The model under review builds one solid part; all positions refer to its coordinate system, in mm. Face numbers are marked on the shaded views. A direction names the side the tool comes from. Round coordinates to 2 decimals unless told otherwise and drop trailing zeros. Order: outer loops, then holes, each group sorted by start corner. A loop starts at its lowest first (then second) coordinate and runs counter-clockwise, first axis right, second up. Notation, with made-up numbers: M -28,-5 L 31,-5 A34 ccw 31,26 Z; hole C -9.5,78 d10. An arc over 180 degrees is marked long. Answer as a JSON object with one key per item and string values. Group by question number.
1. To check wall thickness, follow probe 1 along X at (y, z) = (-214.5, 55); probe 2 along Y at (x, z) = (47, 34.5); probe 3 along X at (y, z) = (-174.5, -2). State the ranges of each line that lie inside material, in increasing order. Write a range as [from, to].
2. Add section B-B on x = 0. State the section outline as (y, z) points, and give its area (3 significant figures).
3. Machinability: for the marked faces 4 and 5, which of the approach directions +Z, -Z, +X, -X, +Y, -Y give a long, thin tool a straight path to every point of the face, cutting with its end or side? Answer none if there is none.
4. Add section A-A on y = -116. State the section outline as (x, z) points.
5. Add section C-C on z = 0. State the section outline as (x, y) points.
6. Add section D-D on x = 47. State the section outline as (y, z) points, and give its area (3 significant figures).
7. Clearance check with flat-ended pins moving along their axes: P1, Ø3, axis at x = 8.5, y = -53.5, coming from the +Z side; P2, Ø2, axis at x = -11.5, y = -177.5, coming from the +Z side; P3, Ø10, axis at x = 18, y = -91.5, coming from the +Z side. State where each tip first meets the part, or that it passes through.
8. Mouldability with a two-part tool opening along X and no side actions: class the marked faces 1, 2 and 3 as released by +X, released by -X, zero draft, split by the parting line, or undercut.
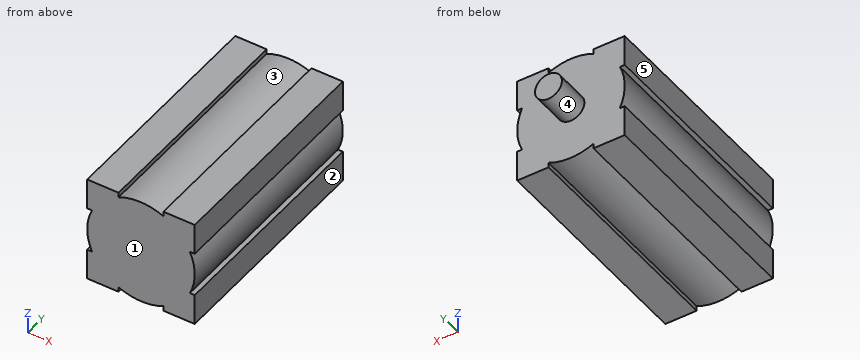
```python
from build123d import *

# Parameters (mm, degrees)
F1_DEPTH = 250
F2_R     = 15
F3_DEPTH = 38


with BuildPart() as f1:
    # F0 (on Front) → F1 (new body)
    with BuildSketch(Plane.XZ):
        with BuildLine():
            Line((-60, 25), (-54.543561, 25))
            ThreePointArc((-54.543561, 25), (-60, 0), (-54.543561, -25))
            Line((-54.543561, -25), (-60, -25))
            Line((-60, -25), (-60, -60))
            Line((-60, -60), (-25, -60))
            Line((-25, -60), (-25, -54.543561))
            ThreePointArc((-25, -54.543561), (0, -60), (25, -54.543561))
            Line((25, -54.543561), (25, -60))
            Line((25, -60), (60, -60))
            Line((60, -60), (60, -25))
            Line((60, -25), (54.543561, -25))
            ThreePointArc((54.543561, -25), (60, 0), (54.543561, 25))
            Line((54.543561, 25), (60, 25))
            Line((60, 25), (60, 60))
            Line((60, 60), (25, 60))
            Line((25, 60), (25, 54.543561))
            ThreePointArc((25, 54.543561), (0, 60), (-25, 54.543561))
            Line((-25, 54.543561), (-25, 60))
            Line((-25, 60), (-60, 60))
            Line((-60, 60), (-60, 25))
        make_face()
    extrude(amount=F1_DEPTH)

    # F2 (on face) → F3 (join)
    with BuildSketch(Plane(origin=(0, 0, 0), x_dir=(-1, 0, 0), z_dir=(0, 1, 0))):
        Circle(F2_R)
    extrude(amount=F3_DEPTH)


solid = f1.part
```
Recorded:
{
 "1": {"probe 1": "x = [-60, -25], [-23.98, 23.98], [25, 60]", "probe 2": "y = [-250, 0]", "probe 3": "x = [-59.97, 59.97]"},
 "2": {"outline": "M -250,-60 L 0,-60 L 0,-15 L 38,-15 L 38,15 L 0,15 L 0,60 L -250,60 Z", "area": "31,100 mm²"},
 "3": {"face 4": "+Y", "face 5": "+Z, -Z, -X, +Y, -Y"},
 "4": {"outline": "M -60,-60 L -25,-60 L -25,-54.54 A60 ccw 25,-54.54 L 25,-60 L 60,-60 L 60,-25 L 54.54,-25 A60 ccw 54.54,25 L 60,25 L 60,60 L 25,60 L 25,54.54 A60 ccw -25,54.54 L -25,60 L -60,60 L -60,25 L -54.54,25 A60 ccw -54.54,-25 L -60,-25 Z"},
 "5": {"outline": "M -60,-250 L 60,-250 L 60,0 L 15,0 L 15,38 L -15,38 L -15,0 L -60,0 Z"},
 "6": {"outline": "M -250,-60 L 0,-60 L 0,60 L -250,60 Z", "area": "30,000 mm²"},
 "7": {"P1": "stops at z = 59.59", "P2": "stops at z = 59.07", "P3": "stops at z = 58.57"},
 "8": {"face 1": "zero draft", "face 2": "released by +X", "face 3": "undercut"}
}
